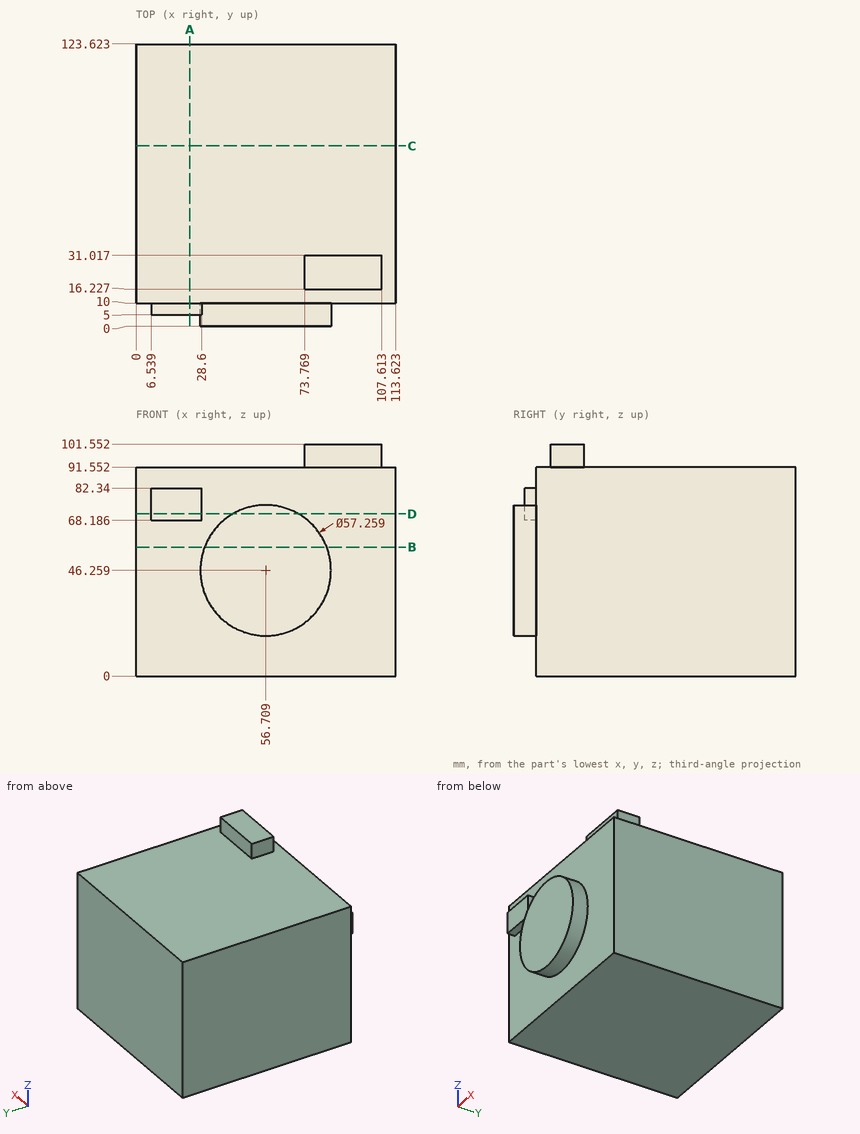
Design review of the part shown in the three views and the two pictorial views. Dimensions are in mm from the part's minimum x, y and z. Round coordinates to 2 decimals unless told otherwise and drop trailing zeros. Order: outer loops, then holes, each group sorted by start corner. A loop starts at its lowest first (then second) coordinate and runs counter-clockwise, first axis right, second up.
Item 1: Add section B-B, the plane z = 56.5. State the section outline as (x, y) points (1 decimal), and give its area (3 significant figures).
Working result:
outline: (0, 10) - (30, 10) - (30, 0) - (83.4, 0) - (83.4, 10) - (113.6, 10) - (113.6, 123.6) - (0, 123.6) - close
area: 13,400 mm2
Item 2: To check wall thickness, follow probe 1 along Y at (x, z) = (75, 96); probe 2 along Y at (x, z) = (14, 65.5); probe 3 along Z at (x, y) = (28, 76). State the ranges of each line that lie inside material, in increasing order.
Working result:
probe 1: y = 16.23 to 31.02
probe 2: y = 10 to 123.62
probe 3: z = 0 to 91.55
Item 3: Add section C-C, the plane y = 79. State the section outline as (x, z) points.
Working result:
outline: (0, 0) - (113.62, 0) - (113.62, 91.55) - (0, 91.55) - close
Item 4: Add section D-D, the plane z = 71. State the section outline as (x, y) points (1 decimal).
Working result:
outline: (0, 10) - (6.5, 10) - (6.5, 5) - (28.6, 5) - (28.6, 10) - (42.3, 10) - (42.3, 0) - (71.1, 0) - (71.1, 10) - (113.6, 10) - (113.6, 123.6) - (0, 123.6) - close
Item 5: Add section A-A, the plane x = 23.5. State the section outline as (y, z) points (1 decimal).
Working result:
outline: (5, 68.2) - (10, 68.2) - (10, 0) - (123.6, 0) - (123.6, 91.6) - (10, 91.6) - (10, 82.3) - (5, 82.3) - close
Item 6: For pin 1 (1.5 mm diameter, centred on y = 7, z = 77.5, fed in from -X); pin 2 (4 mm diameter, centred on x = 33, z = 10, fed in from -Y); pin 3 (5 mm diameter, centred on y = 21.5, z = 98.5, fed in from -X), all flat-tipped, find the tip position at first contact; note any pin that passes through.
Working result:
pin 1: stops at x = 6.54
pin 2: stops at y = 10
pin 3: stops at x = 73.77
